from build123d import *

# Parameters (mm, degrees)
F0_W     = 91.3384
F0_H     = 97.5812673569
F1_DEPTH = 127
F2_W     = 91.3384
F2_H     = 45.5940548778
F3_DEPTH = 63.5
F4_DEPTH = 25.4
F5_W     = 91.3384
F5_H     = 81.4059451222
F6_DEPTH = 78.74


with BuildPart() as f1:
    # F0 (on Top) → F1 (new body)
    with BuildSketch(Plane.XY):
        with Locations((-10.1847631006, -3.307942301)):
            Rectangle(F0_W, F0_H)
    extrude(amount=F1_DEPTH)

    # F2 (on face) → F3 (cut)
    with BuildSketch(Plane.XZ.offset(52.0985759795)):
        with Locations((-10.1847631006, 104.2029725611)):
            Rectangle(F2_W, F2_H)
    extrude(amount=-F3_DEPTH, mode=Mode.SUBTRACT)

    # F4 (add): a face of the model
    f4_faces = [f1.faces().sort_by_distance(p)[0] for p in [
        (-10.1847631006, -52.0985759795, 40.7029725611),
    ]]
    extrude(f4_faces, amount=F4_DEPTH)

    # F5 (on face) → F6 (join)
    with BuildSketch(Plane.XZ.offset(77.4985759795)):
        with Locations((-10.1847631006, 40.7029725611)):
            Rectangle(F5_W, F5_H)
    extrude(amount=F6_DEPTH)


solid = f1.part
Work out the finished part from the listing and answer in its coordinate system (mm). A direction names the side the tool comes from. Round coordinates to 2 decimals unless told otherwise and drop trailing zeros. Loops run counter-clockwise (first coordinate to the right, second up) from the corner with the lowest first, then second, coordinate; pieces in that order, holes last. Notation, with made-up numbers: (-40, -35) -> (-6, -35) arc R29 ccw to (-6, -5) -> close; hole circle Ø4 at (7.25, 78). An arc over 180 degrees is marked (long way). Use one line per item in the form item = value.
(1) Flat-ended cylindrical pins translate along their axes: P1, Ø23, axis at x = 0, z = 106, coming from the -Y side; P2, Ø8, axis at x = 3, y = 8.5, coming from the +Z side. Find the tip coordinate at first contact, or state that the pin passes through.
Answer list:
P1 = 11.4
P2 = 127
(2) Find section B-B on y = -119.5. Give the vertices of the cut face in (x, z), then the cut area to 3 significant figures.
Answer list:
outline = (-55.85, 0) -> (35.48, 0) -> (35.48, 81.41) -> (-55.85, 81.41) -> close
area = 7,440 mm2
(3) A tool of negligible diameter and unlimited length cuts with its end or side. For faces 1 (the flat face through (-55.854, -54, 48)), 2 (the flat face through (-11, 11.401, 105)), from which of +Z, -Z, +X, -X, +Y, -Y can it reach the whole face along a straight path? Write none if from no direction.
Answer list:
face_1 = +Z, -Z, -X, +Y, -Y
face_2 = +Z, +X, -X, -Y
(4) Find section A-A on x = -14. Give the vertices of the cut face in (y, z).
Answer list:
outline = (-156.24, 0) -> (45.48, 0) -> (45.48, 127) -> (11.4, 127) -> (11.4, 81.41) -> (-156.24, 81.41) -> close
(5) Straight lines are drawn through the part: line 1 (Z direction, x = -26.5, y = -110.5); line 2 (Y direction, x = 7.5, z = 101.5). For each, find the intervals that lie inside material, in ascending order.
Answer list:
line_1 = 0 to 81.41
line_2 = 11.4 to 45.48
(6) Find section C-C on z = 109. Give the vertices of the cut face in (x, y), then the cut area to 3 significant figures.
Answer list:
outline = (-55.85, 11.4) -> (35.48, 11.4) -> (35.48, 45.48) -> (-55.85, 45.48) -> close
area = 3,110 mm2
